Part print with two shaded views. Sizes in mm from the minimum x, y, z corner. A direction names the side the tool comes from. Round coordinates to 2 decimals unless told otherwise and drop trailing zeros. Order: outer loops, then holes, each group sorted by start corner. A loop starts at its lowest first (then second) coordinate and runs counter-clockwise, first axis right, second up. Notation, with made-up numbers: (11.25, -13) -> (51.25, -13) arc R34 cw to (51.25, 18) -> close; hole circle Ø11 at (-25.5, 79.25). An arc over 180 degrees is marked (long way). Answer as a JSON object with one key per item and string values.
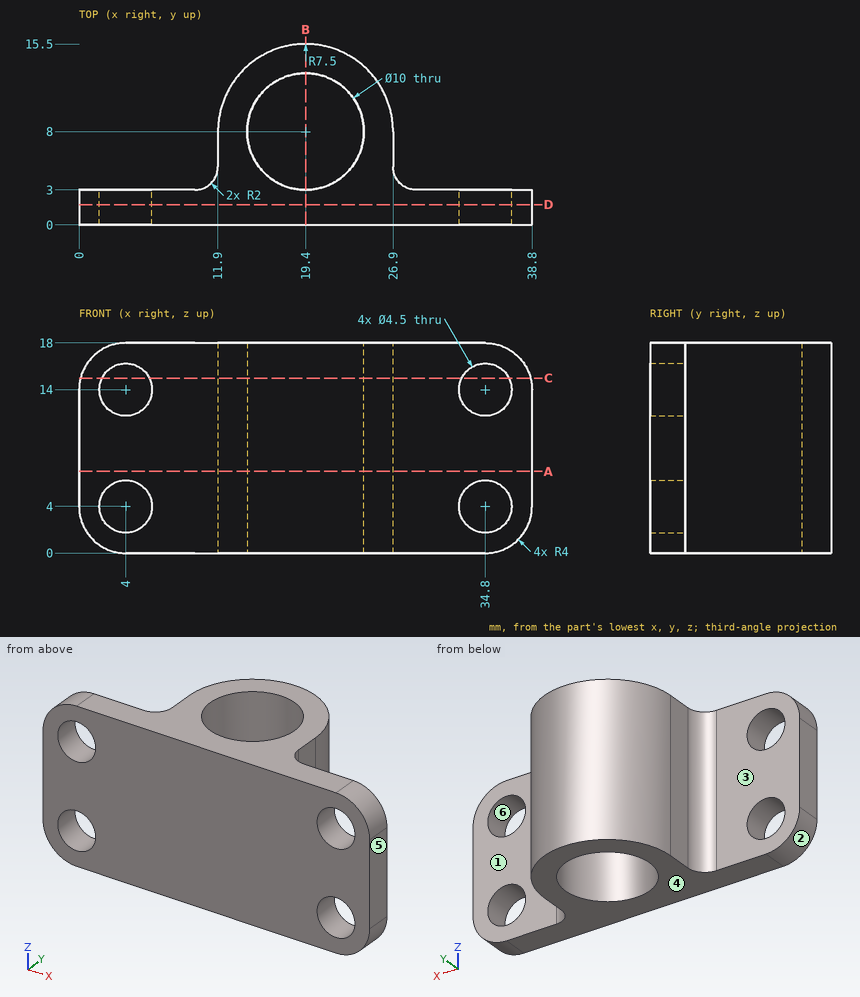
1) Cut at B-B, the plane x = 19.4. Give the cut face in (y, z).
Checked values:
{"outline": "(0, 0) -> (3, 0) -> (3, 18) -> (0, 18) -> close; (13, 0) -> (15.5, 0) -> (15.5, 18) -> (13, 18) -> close"}
2) Probe L1, parallel to Z at x = 34.8, y = 1.9; L2, parallel to X at y = 1.7, z = 14; L3, parallel to Y at x = 19.4, z = 8.5. List the from-to ranges inside material, lowest first. Write a range as from..to.
Checked values:
{"L1": "z = 0..1.75, 6.25..11.75, 16.25..18", "L2": "x = 0..1.75, 6.25..32.55, 37.05..38.8", "L3": "y = 0..3, 13..15.5"}
3) Pull direction X, two halves, no side cores. Call the marked faces 4, 5 and 6: pulls with the +X half, pulls with the -X half, needs draft (parallel to the pull), parting line crosses it, or undercut.
Checked values:
{"face 4": "needs draft", "face 5": "pulls with the +X half", "face 6": "undercut"}
4) Flat gauge pins, fed straight in: pin 1 Ø8 at (y, z) = (2.5, 15) entering from -X; pin 2 Ø0.9 at (y, z) = (6.5, 6) entering from -X; pin 3 Ø5 at (x, z) = (4, 14) entering from +Y; pin 4 Ø3.5 at (x, z) = (4, 4) entering from -Y (3 decimals). Where does each tip first touch, or does it go through?
Checked values:
{"pin 1": "stops at x = 0", "pin 2": "stops at x = 11.9", "pin 3": "stops at y = 3", "pin 4": "passes through"}
5) Cut at A-A, the plane z = 7. Give the cut face in (x, y).
Checked values:
{"outline": "(0, 0) -> (38.8, 0) -> (38.8, 3) -> (28.9, 3) arc R2 cw to (26.9, 5) -> (26.9, 8) arc R7.5 ccw to (11.9, 8) -> (11.9, 5) arc R2 cw to (9.9, 3) -> (0, 3) -> close; hole circle Ø10 at (19.4, 8)"}
6) Which spindle directions (+Z, -Z, +X, -X, +Y, -Y) get a long thin tool onto all of the face, cutting with end or side? Do the marked faces 1, 2 and 3. Say none if no direction does.
Checked values:
{"face 1": "+Z, -Z, +X, +Y", "face 2": "-Z, -X, +Y, -Y", "face 3": "+Z, -Z, -X, +Y"}
7) Cut at D-D, the plane y = 1.75. Give the cut face in (x, z), plus the area to 3 significant figures.
Checked values:
{"outline": "(0, 4) arc R4 ccw to (4, 0) -> (34.8, 0) arc R4 ccw to (38.8, 4) -> (38.8, 14) arc R4 ccw to (34.8, 18) -> (4, 18) arc R4 ccw to (0, 14) -> close; hole circle Ø4.5 at (4, 4); hole circle Ø4.5 at (4, 14); hole circle Ø4.5 at (34.8, 4); hole circle Ø4.5 at (34.8, 14)", "area": "621 mm²"}
8) Cut at C-C, the plane z = 15. Give the cut face in (x, y), plus the area to 3 significant figures.
Checked values:
{"outline": "(0.13, 0) -> (1.98, 0) -> (1.98, 3) -> (0.13, 3) -> close; (6.02, 0) -> (32.78, 0) -> (32.78, 3) -> (28.9, 3) arc R2 cw to (26.9, 5) -> (26.9, 8) arc R7.5 ccw to (11.9, 8) -> (11.9, 5) arc R2 cw to (9.9, 3) -> (6.02, 3) -> close; (36.82, 0) -> (38.67, 0) -> (38.67, 3) -> (36.82, 3) -> close; hole circle Ø10 at (19.4, 8)", "area": "178 mm²"}
